The drawing under review shows one solid part. Ordinate dimensions are in mm from its lowest x, y, z. Give positions to 0.01 mm unless a question says otherwise; leave off trailing zeros. Loops run counter-clockwise (first coordinate to the right, second up) from the corner with the lowest first, then second, coordinate; pieces in that order, holes last.
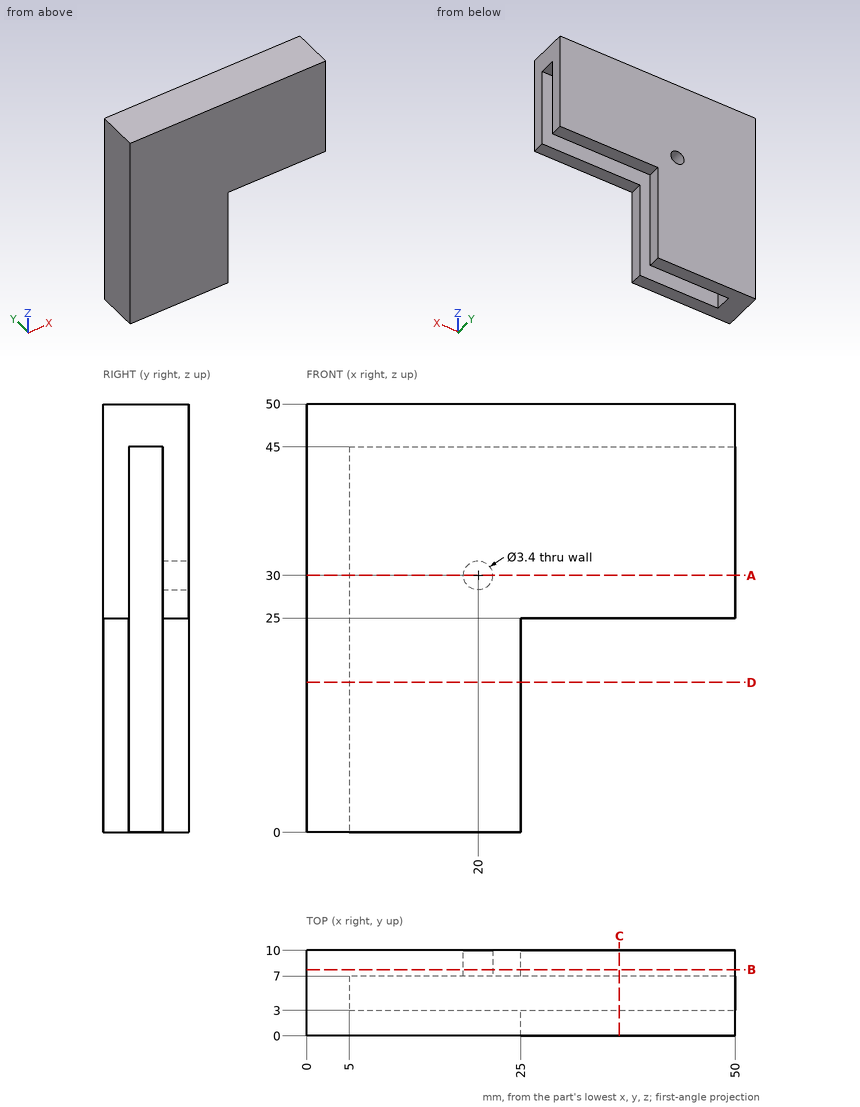
Item 1: Take a section at A-A on z = 30. Give the boundary of the cut face in (x, y).
Answer:
outline: (0, 0) - (50, 0) - (50, 3) - (5, 3) - (5, 7) - (18.3, 7) - (18.3, 10) - (0, 10) - close; (21.7, 7) - (50, 7) - (50, 10) - (21.7, 10) - close
Item 2: Take a section at B-B on y = 7.75. Give the boundary of the cut face in (x, z).
Answer:
outline: (0, 0) - (25, 0) - (25, 25) - (50, 25) - (50, 50) - (0, 50) - close; hole circle Ø3.4 at (20, 30)
Item 3: Take a section at C-C on x = 36.5. Give the boundary of the cut face in (y, z).
Answer:
outline: (0, 25) - (3, 25) - (3, 45) - (7, 45) - (7, 25) - (10, 25) - (10, 50) - (0, 50) - close
Item 4: Take a section at D-D on z = 17.5. Give the boundary of the cut face in (x, y), and give its area (3 significant figures).
Answer:
outline: (0, 0) - (25, 0) - (25, 3) - (5, 3) - (5, 7) - (25, 7) - (25, 10) - (0, 10) - close
area: 170 mm2
Item 5: Clearance check with flat-ended pins moving along their axes: pin 1 Ø0.9 at (y, z) = (9, 18) entering from +X; pin 2 Ø1.2 at (y, z) = (4, 31.5) entering from +X; pin 3 Ø2.5 at (x, y) = (39.5, 8.5) entering from -Z. State where each tip first meets the part, or that it passes through.
Answer:
pin 1: stops at x = 25
pin 2: stops at x = 5
pin 3: stops at z = 25
Item 6: For L1, parallel to Z at x = 20, y = 7.6; L2, parallel to X at y = 7.8, z = 30; L3, parallel to Y at x = 29, z = 31, list the stretches that pass through material, from the lowest coordinate up.
Answer:
L1: z = 0 to 28.3, 31.7 to 50
L2: x = 0 to 18.3, 21.7 to 50
L3: y = 0 to 3, 7 to 10
